Input: part model. Units: mm. Frame: model coordinates. A direction names the side the tool comes from. Coordinates: 2 decimals unless noted, no trailing zeros. Loops run counter-clockwise (first coordinate to the right, second up) from the corner with the lowest first, then second, coordinate; pieces in that order, holes last. Notation, with made-up numbers: (-1.75, 78.25) -> (31.25, 78.25) arc R15 cw to (31.25, 103.25) -> close; hole circle Ø6 at (44, 77.5). An arc over 180 degrees is marked (long way). Answer as a JSON object with one key per item and string values.
from build123d import *

# Parameters (mm, degrees)
FILLET1_R = 0.508


with BuildPart() as part:
    # Sketch1 → Revolve1 (revolve)
    with BuildSketch(Plane.YZ, mode=Mode.PRIVATE) as revolve1_sk:
        Polygon((0, 3.000000096), (-6.000000192, 3.000000096), (-6.000000192, 7.112), (-5.00000016, 7.112), (-5.00000016, 5.588), (-1.000000032, 5.588), (-1.000000032, 7.112), (0, 7.112), align=None)
    revolve(revolve1_sk.sketch.rotate(Axis((0, -39.041586513, 0), (0, 1, 0)), 180), axis=Axis((0, -39.041586513, 0), (0, 1, 0)))

    # Fillet1
    fillet1_edges = [part.edges().sort_by_distance(p)[0] for p in [
        (0, -1.000000032, 7.112),
        (0, -5.00000016, 7.112),
    ]]
    fillet(fillet1_edges, radius=FILLET1_R)


solid = part.part
1. Access query for faces 1 (the face through (1, 0, -3)), 2 (the face through (-3, -5, 5)). Directions: +Z, -Z, +X, -X, +Y, -Y. A direction counts if a zero-diameter tool reaches every point of the face in a straight line with its end or side. Return the directions, or none.
Reply:
{"face 1": "+Z, -Z, +X, -X, +Y", "face 2": "none"}
2. Section query C-C (y = -4). Return loops of the section in (x, z), plus the area to 3 significant figures.
Reply:
{"outline": "circle Ø11.18 at (0, 0); hole circle Ø6 at (0, 0)", "area": "69.8 mm2"}
3. Pin query (flat end, axial travel): P1, Ø3, axis at x = 4.5, y = -1.5, coming from the +Z side. Return the tip coordinate at first contact, or that it passes through.
Reply:
{"P1": "stops at z = 6.29"}
4. Line query: line 1 along Y through (x, z) = (6, 1); line 2 along X through (y, z) = (-3.5, 0); line 3 along Z through (x, y) = (-0.5, -3.25). Output: solid intervals per line, ascending.
Reply:
{"line 1": "y = -6 to -5, -1 to 0", "line 2": "x = -5.59 to -3, 3 to 5.59", "line 3": "z = -5.57 to -2.96, 2.96 to 5.57"}
5. Section query B-B (x = 0). Return loops of the section in (y, z).
Reply:
{"outline": "(-6, -7.11) -> (-5.51, -7.11) arc R0.51 ccw to (-5, -6.6) -> (-5, -5.59) -> (-1, -5.59) -> (-1, -6.6) arc R0.51 ccw to (-0.49, -7.11) -> (0, -7.11) -> (0, -3) -> (-6, -3) -> close; (-6, 3) -> (0, 3) -> (0, 7.11) -> (-0.49, 7.11) arc R0.51 ccw to (-1, 6.6) -> (-1, 5.59) -> (-5, 5.59) -> (-5, 6.6) arc R0.51 ccw to (-5.51, 7.11) -> (-6, 7.11) -> close"}
6. Mould query, pull axis X, two halves, no side actions, for faces 3 (the face through (2.93, -3.04, 0.65)), 4 (the face through (3.4, -2.972, 4.434)), 5 (the face through (1, -6, 3)). Classes: pulls with the +X half, pulls with the -X half, needs draft (parallel to the pull), parting line crosses it, or undercut.
Reply:
{"face 3": "undercut", "face 4": "parting line crosses it", "face 5": "needs draft"}
7. Section query A-A (z = 0). Return loops of the section in (x, y), plus the area to 3 significant figures.
Reply:
{"outline": "(-7.11, -6) -> (-3, -6) -> (-3, 0) -> (-7.11, 0) -> (-7.11, -0.49) arc R0.51 ccw to (-6.6, -1) -> (-5.59, -1) -> (-5.59, -5) -> (-6.6, -5) arc R0.51 ccw to (-7.11, -5.51) -> close; (3, -6) -> (7.11, -6) -> (7.11, -5.51) arc R0.51 ccw to (6.6, -5) -> (5.59, -5) -> (5.59, -1) -> (6.6, -1) arc R0.51 ccw to (7.11, -0.49) -> (7.11, 0) -> (3, 0) -> close", "area": "36.9 mm2"}
8. Section query D-D (y = -0.75). Return loops of the section in (x, z).
Reply:
{"outline": "circle Ø14.08 at (0, 0); hole circle Ø6 at (0, 0)"}
